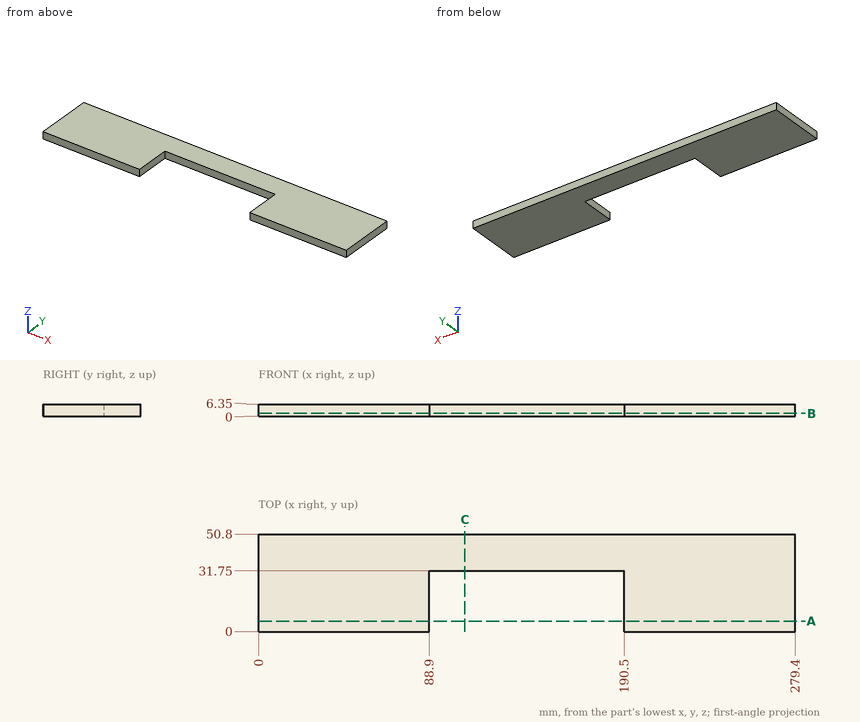
The drawing under review shows one solid part. Ordinate dimensions are in mm from its lowest x, y, z. Round coordinates to 2 decimals unless told otherwise and drop trailing zeros. Write each loop counter-clockwise with the first axis right and the second up, starting at its lowest first coordinate (ties: lowest second). Pieces come first, ordered by that corner, then holes. Notation, with made-up numbers: (15.25, 87) - (40.25, 87) arc R14 cw to (40.25, 106) - close; hole circle Ø2 at (51.5, -32). An arc over 180 degrees is marked (long way). Use one line per item in the form item = value.
Q1. For line 1 (X direction, y = 5.5, z = 2.75); line 2 (Y direction, x = 160.5, z = 4.5), list the stretches that pass through material, from the lowest coordinate up. Write a range as [from, to].
Answer key:
line_1 = [0, 88.9], [190.5, 279.4]
line_2 = [31.75, 50.8]
Q2. Consider section B-B (z = 1.5). State the section outline as (x, y) points.
Answer key:
outline = (0, 0) - (88.9, 0) - (88.9, 31.75) - (190.5, 31.75) - (190.5, 0) - (279.4, 0) - (279.4, 50.8) - (0, 50.8) - close
Q3. Consider section A-A (y = 5.5). State the section outline as (x, z) points, and give its area (3 significant figures).
Answer key:
outline = (0, 0) - (88.9, 0) - (88.9, 6.35) - (0, 6.35) - close; (190.5, 0) - (279.4, 0) - (279.4, 6.35) - (190.5, 6.35) - close
area = 1,130 mm2
Q4. Consider section C-C (x = 107.5). State the section outline as (y, z) points.
Answer key:
outline = (31.75, 0) - (50.8, 0) - (50.8, 6.35) - (31.75, 6.35) - close
